```python
from build123d import *

# Parameters (mm, degrees)
SKETCH1_R           = 1.7
SKETCH1_R_2         = 1.75
BOSS_EXTRUDE1_DEPTH = 2.75
SKETCH2_R           = 4.5
SKETCH2_R_2         = 3.25
BOSS_EXTRUDE2_DEPTH = 3.2
BOSS_EXTRUDE3_DEPTH = 3.2
CIRPATTERN1_COUNT   = 28
SKETCH4_R           = 4.5
SKETCH4_R_2         = 3.5
SKETCH4_R_3         = 3
SKETCH4_R_4         = 1.7
CUT_EXTRUDE1_DEPTH  = 1
FILLET1_R           = 0.25
FILLET2_R           = 0.2


with BuildPart() as part:
    # Sketch1 → Boss-Extrude1 (new body)
    with BuildSketch(Plane(origin=(0, 0, 0), x_dir=(1, 0, 0), z_dir=(0, 1, 0))):
        with BuildLine():
            Line((-30, 4.082414086), (-4.589117562, 4.95))
            ThreePointArc((-4.589117562, 4.95), (0, 6.75), (4.589117562, 4.95))
            ThreePointArc((4.589117562, 4.95), (6.639474696, 0), (4.589117562, -4.95))
            ThreePointArc((4.589117562, -4.95), (0, -6.75), (-4.589117562, -4.95))
            Line((-4.589117562, -4.95), (-30, -4.082414086))
            ThreePointArc((-30, -4.082414086), (-34.082414086, 0), (-30, 4.082414086))
        make_face()
        with Locations(Location((0, 0, 0), (0, 0, 270))):
            Circle(SKETCH1_R, mode=Mode.SUBTRACT)
        with Locations(Location((-30, 0, 0), (0, 0, 270))):
            Circle(SKETCH1_R_2, mode=Mode.SUBTRACT)
    extrude(amount=BOSS_EXTRUDE1_DEPTH)

    # Sketch2 → Boss-Extrude2 (add)
    with BuildSketch(Plane(origin=(0, 2.75, 0), x_dir=(1, 0, 0), z_dir=(0, 1, 0))):
        with Locations(Location((0, 0, 0), (0, 0, 270))):
            Circle(SKETCH2_R)
        with Locations(Location((0, 0, 0), (0, 0, 270))):
            Circle(SKETCH2_R_2, mode=Mode.SUBTRACT)
    extrude(amount=BOSS_EXTRUDE2_DEPTH)

    # Sketch3 → Boss-Extrude3 (add)
    with BuildSketch(Plane(origin=(0, 5.95, 0), x_dir=(1, 0, 0), z_dir=(0, 1, 0))):
        Polygon((-0.3, 3.25), (0.3, 3.25), (0, 2.85), align=None)
    boss_extrude3 = extrude(amount=-BOSS_EXTRUDE3_DEPTH)

    # CirPattern1: Boss-Extrude3 ×28 about axis
    cirpattern1_axis = Axis((0, 0, 0), (0, 1, 0))
    for i in range(1, CIRPATTERN1_COUNT):
        add(boss_extrude3.rotate(cirpattern1_axis, i * 360 / CIRPATTERN1_COUNT))

    # Sketch4 → Cut-Extrude1 (cut)
    # profile 1 of 2: a face of its own
    with BuildSketch(Plane.XZ):
        with Locations(Location((0, 0, 0), (0, 0, 90))):
            Circle(SKETCH4_R)
        with Locations(Location((0, 0, 0), (0, 0, 270))):
            Circle(SKETCH4_R_2, mode=Mode.SUBTRACT)
    # profile 2 of 2: a face of its own
    with BuildSketch(Plane.XZ):
        with Locations(Location((0, 0, 0), (0, 0, 270))):
            Circle(SKETCH4_R_3)
        with Locations(Location((0, 0, 0), (0, 0, 270))):
            Circle(SKETCH4_R_4, mode=Mode.SUBTRACT)
    extrude(amount=-CUT_EXTRUDE1_DEPTH, mode=Mode.SUBTRACT)

    # Fillet1
    fillet1_edges = [part.edges().sort_by_distance(p)[0] for p in [
        (0, 0, 3.5),
        (0, 0, -4.5),
        (0, 0, 3),
    ]]
    fillet(fillet1_edges, radius=FILLET1_R - 0.0001)  # a hair under: the kernel refuses the full size

    # Fillet2
    fillet2_edges = [part.edges().sort_by_distance(p)[0] for p in [
        (0, 5.95, -4.5),
    ]]
    fillet(fillet2_edges, radius=FILLET2_R)


solid = part.part
```
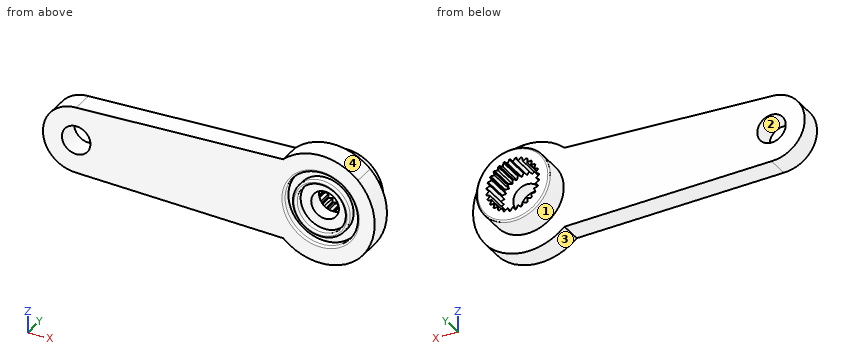
Design review of the part built by this model. Coordinates are the model's own, in mm. Face numbers are marked on the shaded views. Give positions to 0.01 mm unless a question says otherwise; leave off trailing zeros. Write each loop counter-clockwise with the first axis right and the second up, starting at its lowest first coordinate (ties: lowest second). Pieces come first, ordered by that corner, then holes. Notation, with made-up numbers: (-4, 22) -> (55, 22) arc R13 ccw to (55, 39) -> close; hole circle Ø1 at (13.5, 84). An arc over 180 degrees is marked (long way). Answer in a Markdown table with one row per item.
(1) To check wall thickness, follow probe 1 along X at (y, z) = (1.9, 0); probe 2 along X at (y, z) = (0.45, 0); probe 3 along Y at (x, z) = (-2, -3.5). State the ranges of each line that lie inside material, in increasing order.
Results:
| item | result |
|---|---|
| probe 1 | -34.08 to -31.75, -28.25 to -1.7, 1.7 to 6.64 |
| probe 2 | -34.08 to -31.75, -28.25 to -4.5, -3.5 to -3, 3 to 3.5, 4.5 to 6.64 |
| probe 3 | 1 to 5.95 |
(2) Consider section A-A (x = -29). State the section outline as (y, z) points, then the cut area to 3 significant figures.
Results:
| item | result |
|---|---|
| outline | (0, -4.12) -> (2.75, -4.12) -> (2.75, -1.44) -> (0, -1.44) -> close; (0, 1.44) -> (2.75, 1.44) -> (2.75, 4.12) -> (0, 4.12) -> close |
| area | 14.7 mm2 |
(3) Mouldability with a two-part tool opening along Z and no side actions: class the marked faces 1, 2, 3 and 4 as +Z half, -Z half, draft (parallel to the pull), parting line (faces both ways), or undercut.
Results:
| item | result |
|---|---|
| face 1 | parting line |
| face 2 | undercut |
| face 3 | -Z half |
| face 4 | +Z half |
(4) Consider section B-B (x = -12). State the section outline as (y, z) points, then the cut area to 3 significant figures.
Results:
| item | result |
|---|---|
| outline | (0, -4.7) -> (2.75, -4.7) -> (2.75, 4.7) -> (0, 4.7) -> close |
| area | 25.8 mm2 |
(5) Clearance check with flat-ended pins moving along their axes: pin 1 (6 mm diameter, centred on x = -15, z = -4, fed in from -Y); pin 2 (3 mm diameter, centred on x = -3, z = 5, fed in from +Y); pin 3 (3 mm diameter, centred on x = 1, z = 1, fed in from -Y); pin 4 (3.5 mm diameter, centred on x = 0, z = 0, fed in from +Y). State where each tip first meets the part, or that it passes through.
Results:
| item | result |
|---|---|
| pin 1 | y = 0 |
| pin 2 | y = 5.95 |
| pin 3 | y = 1 |
| pin 4 | y = 2.75 |
(6) Consider section C-C (x = -24). State the section outline as (y, z) points, then the cut area to 3 significant figures.
Results:
| item | result |
|---|---|
| outline | (0, -4.29) -> (2.75, -4.29) -> (2.75, 4.29) -> (0, 4.29) -> close |
| area | 23.6 mm2 |
